Read the model definition and answer for the solid it produces. Units are mm, in the model's axes. Face numbers are marked on the shaded views. Give positions to 0.01 mm unless a question says otherwise; leave off trailing zeros. Order: outer loops, then holes, each group sorted by start corner. A loop starts at its lowest first (then second) coordinate and runs counter-clockwise, first axis right, second up. Notation, with made-up numbers: (-4, 4.25) - (39, 4.25) arc R23 cw to (39, 24.25) - close; hole circle Ø10 at (35, -39). An arc over 180 degrees is marked (long way). Return JSON: item names as keys, results as strings.
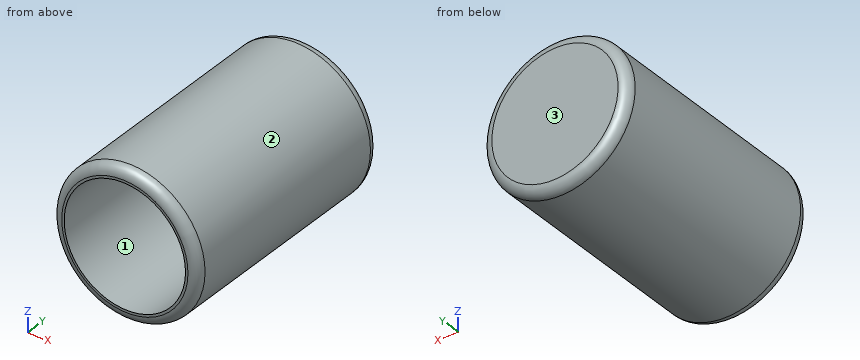
```python
from build123d import *

# Parameters (mm, degrees)
F0_R     = 38.1
F0_R_2   = 31.75
F1_DEPTH = 123.825
F2_R     = 31.75
F3_DEPTH = 9.525
F4_R     = 5.08


with BuildPart() as f1:
    # F0 (on Front) → F1 (new body)
    with BuildSketch(Plane.XZ):
        Circle(F0_R)
        Circle(F0_R_2, mode=Mode.SUBTRACT)
    extrude(amount=F1_DEPTH)

    # F2 (on Front) → F3 (join)
    with BuildSketch(Plane.XZ):
        Circle(F2_R)
    extrude(amount=F3_DEPTH)

    # F4
    f4_edges = [f1.edges().sort_by_distance(p)[0] for p in [
        (-38.1, -123.825, 0),
        (38.1, -61.9125, 0),
        (-38.1, 0, 0),
    ]]
    fillet(f4_edges, radius=F4_R)


solid = f1.part
```
Q1. A cutting plane is placed at B-B (z = 0). Write down the section's boundary in (x, y) (3 decimals), and give its area (3 significant figures).
Values:
{"outline": "(-38.1, -118.745) arc R5.08 ccw to (-33.02, -123.825) - (-31.75, -123.825) - (-31.75, -9.525) - (31.75, -9.525) - (31.75, -123.825) - (33.02, -123.825) arc R5.08 ccw to (38.1, -118.745) - (38.1, -5.08) arc R5.08 ccw to (33.02, 0) - (-33.02, 0) arc R5.08 ccw to (-38.1, -5.08) - close", "area": "2,160 mm²"}
Q2. Given pin 1 (3 mm diameter, centred on x = -4, z = 16.5, fed in from -Y) (3 decimals); pin 2 (5 mm diameter, centred on x = -18, y = -76, fed in from +Z); pin 3 (2 mm diameter, centred on y = -54, z = 16, fed in from -X), each flat-ended and moving along its own axis, determine where each tip first touches the part or whether it passes through.
Values:
{"pin 1": "stops at y = -9.525", "pin 2": "stops at z = 34.8", "pin 3": "stops at x = -35.02"}
Q3. Consider L1, parallel to Z at x = 0, y = -61; L2, parallel to Y at x = -1, z = -22.5 (3 decimals); L3, parallel to X at y = -90, z = 22. Determine where each line is inside the solid, lowest interval first.
Values:
{"L1": "z = -38.1 to -31.75, 31.75 to 38.1", "L2": "y = -9.525 to 0", "L3": "x = -31.11 to -22.89, 22.89 to 31.11"}
Q4. Determine the mould class of the marked faces 1, 2 and 3 for opening direction X: released by +X, released by -X, zero draft, split by the parting line, or undercut.
Values:
{"face 1": "undercut", "face 2": "split by the parting line", "face 3": "zero draft"}
Q5. A cutting plane is placed at C-C (y = -116). Write down the section's boundary in (x, z), and give its area (3 significant figures).
Values:
{"outline": "circle Ø76.2 at (0, 0); hole circle Ø63.5 at (0, 0)", "area": "1,390 mm²"}
Q6. A cutting plane is placed at A-A (x = 0). Write down the section's boundary in (y, z) (3 decimals), and give its area (3 significant figures).
Values:
{"outline": "(-123.825, -33.02) arc R5.08 ccw to (-118.745, -38.1) - (-5.08, -38.1) arc R5.08 ccw to (0, -33.02) - (0, 33.02) arc R5.08 ccw to (-5.08, 38.1) - (-118.745, 38.1) arc R5.08 ccw to (-123.825, 33.02) - (-123.825, 31.75) - (-9.525, 31.75) - (-9.525, -31.75) - (-123.825, -31.75) - close", "area": "2,160 mm²"}
